Work out the finished part from the listing and answer in its coordinate system (mm). Give positions to 0.01 mm unless a question says otherwise; leave off trailing zeros. Order: outer loops, then holes, each group sorted by start corner. A loop starts at its lowest first (then second) coordinate and runs counter-clockwise, first axis right, second up. Notation, with made-up numbers: (18.25, -23) -> (72.25, -23) arc R20 cw to (72.25, 16) -> close; hole circle Ø4 at (28, 86.25). An arc over 180 degrees is marked (long way). Answer as CSV lines item,"result". Start each with the question number.
1. A cutting plane is placed at C-C (x = 42.5). Give the vertices of the cut face in (y, z).
2. Find the intervals of material crossed by L1, parallel to Z at x = 41, y = 1.7; L2, parallel to X at y = 2.95, z = -511; L3, parallel to Z at x = 191.5, y = 1.8, in increasing order.
3. A cutting plane is placed at B-B (y = 2.25). Give the vertices of the cut face in (x, z).
4. A cutting plane is placed at A-A (z = -113.5). Give the vertices of the cut face in (x, y), then the cut area to 4 significant figures.
from build123d import *

# Parameters (mm, degrees)
SKETCH1_W           = 440
SKETCH1_H           = 668.38
BOSS_EXTRUDE1_DEPTH = 3
CUT_EXTRUDE1_DEPTH  = 4


with BuildPart() as part:
    # Sketch1 → Boss-Extrude1 (new body)
    with BuildSketch(Plane(origin=(0, 0, 0), x_dir=(1, 0, 0), z_dir=(0, 1, 0))):
        with Locations((220, 334.19)):
            Rectangle(SKETCH1_W, SKETCH1_H)
    extrude(amount=BOSS_EXTRUDE1_DEPTH)

    # Sketch2 → Cut-Extrude1 (cut, through all)
    with BuildSketch(Plane.XZ):
        Polygon((240, 0), (0, -240), (0, 0), align=None)
        Polygon((0, -428.38), (240, -668.38), (0, -668.38), align=None)
    extrude(amount=-CUT_EXTRUDE1_DEPTH, mode=Mode.SUBTRACT)


solid = part.part
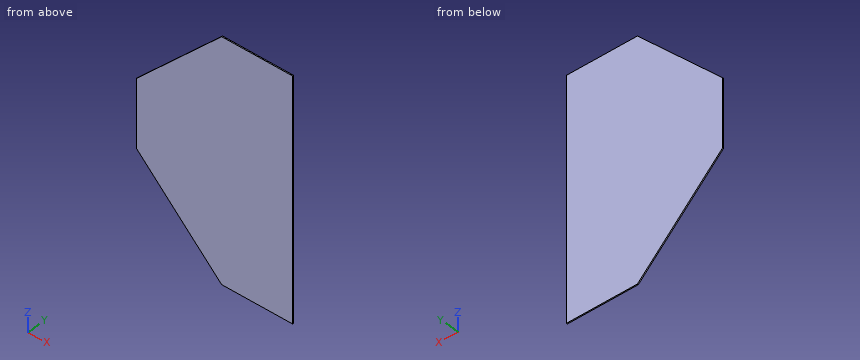
Answer sheet:
1,outline,"(0, -470.88) -> (3, -470.88) -> (3, -197.5) -> (0, -197.5) -> close"
2,L1,"z = -469.38 to -199"
2,L2,"x = 82.62 to 440"
2,L3,"z = -619.88 to -48.5"
3,outline,"(0, -428.38) -> (240, -668.38) -> (440, -668.38) -> (440, 0) -> (240, 0) -> (0, -240) -> close"
4,outline,"(126.5, 0) -> (440, 0) -> (440, 3) -> (126.5, 3) -> close"
4,area,"940.5 mm^2"
